Source: CAD feature listing. Evaluate the final solid. Frame: model axes, mm. Face numbers are marked on the shaded views. Coordinates: 2 decimals unless noted, no trailing zeros. Order: outer loops, then holes, each group sorted by start corner. A loop starts at its lowest first (then second) coordinate and runs counter-clockwise, first axis right, second up. Notation, with made-up numbers: (61, 17.25) -> (113, 17.25) arc R26 ccw to (113, 52.25) -> close; hole circle Ø6 at (-7, 54.25). An arc over 180 degrees is marked (long way). Put each result on its own line as item: value.
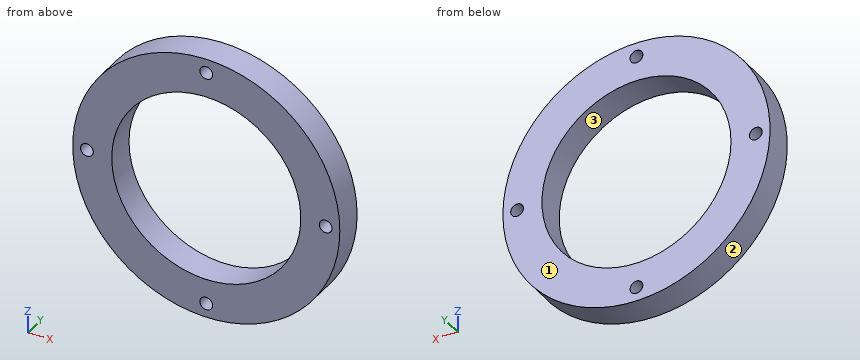
from build123d import *

# Parameters (mm, degrees)
SKETCH2_R               = 45
BOSS_EXTRUDE1_DEPTH     = 10
SKETCH7_R               = 31.85
CUT_EXTRUDE1_DEPTH      = 1
CUT_EXTRUDE1_DEPTH_BACK = 11
SKETCH8_R               = 2.15
CUT_EXTRUDE2_DEPTH      = 11


with BuildPart() as part:
    # Sketch2 → Boss-Extrude1 (new body)
    with BuildSketch(Plane(origin=(0, 0, 0), x_dir=(1, 0, 0), z_dir=(0, 1, 0))):
        Circle(SKETCH2_R)
    extrude(amount=-BOSS_EXTRUDE1_DEPTH)

    # Sketch7 → Cut-Extrude1 (cut, two sides)
    with BuildSketch(Plane(origin=(0, -10, 0), x_dir=(-1, 0, 0), z_dir=(0, -1, 0))) as cut_extrude1_sk:
        Circle(SKETCH7_R)
    extrude(amount=CUT_EXTRUDE1_DEPTH, mode=Mode.SUBTRACT)
    extrude(cut_extrude1_sk.sketch, amount=-CUT_EXTRUDE1_DEPTH_BACK, mode=Mode.SUBTRACT)

    # Sketch8 → Cut-Extrude2 (cut, through all)
    with BuildSketch(Plane.XZ.offset(10)):
        with Locations((-40.22, 0)):
            Circle(SKETCH8_R)
        with Locations((0, -40.22)):
            Circle(SKETCH8_R)
        with Locations((0, 40.22)):
            Circle(SKETCH8_R)
        with Locations((40.22, 0)):
            Circle(SKETCH8_R)
    extrude(amount=-CUT_EXTRUDE2_DEPTH, mode=Mode.SUBTRACT)


solid = part.part
1. Pull-direction query (Z, two-part tool) for the marked faces 1, 2 and 3; classes: pulls with the +Z half, pulls with the -Z half, needs draft (parallel to the pull), parting line crosses it, or undercut.
Numbers:
face 1: needs draft
face 2: parting line crosses it
face 3: undercut
2. First-contact query: pin 1 (1.5 mm diameter, centred on x = 14, y = -8, fed in from +Z); pin 2 (4 mm diameter, centred on y = -1.5, z = -32, fed in from +X); pin 3 (5 mm diameter, centred on x = 0, z = 40.22, fed in from +Y); pin 4 (2 mm diameter, centred on x = 10, y = -8, fed in from +Z). Flat tips, straight axial feed; report the tip coordinate or a pass-through.
Numbers:
pin 1: stops at z = 43.01
pin 2: stops at x = 33.54
pin 3: stops at y = 0
pin 4: stops at z = 44.09
3. Cut plane D-D on x = -33. Output: boundary loops of the cut face in (y, z), plus the area to 3 significant figures.
Numbers:
outline: (-10, -30.59) -> (0, -30.59) -> (0, 30.59) -> (-10, 30.59) -> close
area: 612 mm2
4. Cut plane A-A on x = -18.5. Output: boundary loops of the cut face in (y, z), plus the area to 3 significant figures.
Numbers:
outline: (-10, -41.02) -> (0, -41.02) -> (0, -25.93) -> (-10, -25.93) -> close; (-10, 25.93) -> (0, 25.93) -> (0, 41.02) -> (-10, 41.02) -> close
area: 302 mm2
5. Cut plane C-C on y = -7. Output: boundary loops of the cut face in (x, z).
Numbers:
outline: circle Ø90 at (0, 0); hole circle Ø4.3 at (-40.22, 0); hole circle Ø63.7 at (0, 0); hole circle Ø4.3 at (0, -40.22); hole circle Ø4.3 at (0, 40.22); hole circle Ø4.3 at (40.22, 0)
6. Cut plane B-B on z = 27.5. Output: boundary loops of the cut face in (x, y), plus the area to 3 significant figures.
Numbers:
outline: (-35.62, -10) -> (-16.07, -10) -> (-16.07, 0) -> (-35.62, 0) -> close; (16.07, -10) -> (35.62, -10) -> (35.62, 0) -> (16.07, 0) -> close
area: 391 mm2
7. Ray query, line 1 along Z through (x, y) = (0, -7.25); line 2 along X through (y, z) = (-1, 23); line 3 along Z through (x, y) = (28.5, -7). Return the intervals inside material, ascending.
Numbers:
line 1: z = -45 to -42.37, -38.07 to -31.85, 31.85 to 38.07, 42.37 to 45
line 2: x = -38.68 to -22.03, 22.03 to 38.68
line 3: z = -34.82 to -14.22, 14.22 to 34.82
